Check sheet for the modelled part. Datum: model origin and axes. Units: mm. Face numbers are marked on the shaded views. Round coordinates to 2 decimals unless told otherwise and drop trailing zeros. Loops run counter-clockwise (first coordinate to the right, second up) from the corner with the lowest first, then second, coordinate; pieces in that order, holes last. Notation, with made-up numbers: (8.25, 65.25) - (64.25, 65.25) arc R33 ccw to (64.25, 96.25) - close; hole circle Ø9 at (44.5, -22.5). An arc over 180 degrees is marked (long way). Answer in a Markdown table with one row per item. Add a question column.
(1) Gauge pin test, flat ends, axial feed: pin 1 (3 mm diameter, centred on x = -10, y = 0, fed in from -Z); pin 2 (4.5 mm diameter, centred on x = 13, z = 21, fed in from +Y); pin 3 (10 mm diameter, centred on x = -2.5, z = 12.5, fed in from +Y). Record the tip position at first contact, or that the pin passes through.
(2) Cross-section at A-A on x = 13. Enter the section's corners in (y, z), then the cut area to 3 significant figures.
(3) Thickness scan on line 1 along Z through (x, y) = (-13, -4.05); line 2 along X through (y, z) = (-4.8, 9); line 3 along Z through (x, y) = (-13, -3.95). Record the ranges inside material, lowest first.
(4) Mould release check, pull along Y, two halves, no side actions. Record for the marked faces 1, 2, 3 and 4: +Y half, -Y half, draft (parallel to the pull), parting line (faces both ways), or undercut.
(5) Cross-section at C-C on z = 20.5. Enter the section's corners in (x, y).
(6) Cross-section at D-D on x = -2.5. Enter the section's corners in (y, z).
(7) Cross-section at B-B on y = 0. Enter the section's corners in (x, z), then the cut area to 3 significant figures.
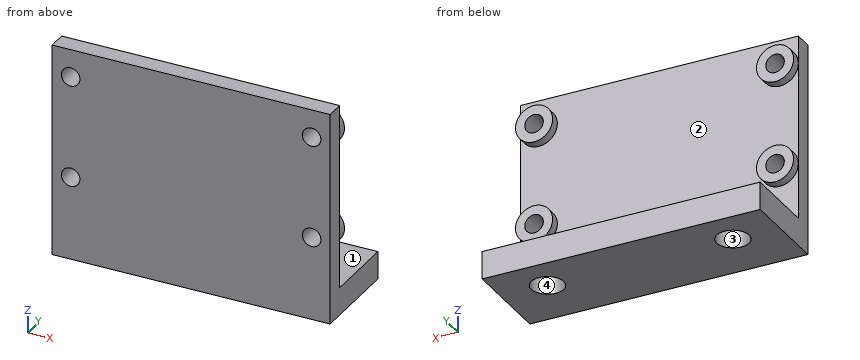
Autodesk Inventor part; units mm, degrees
ref_plane "YZ Plane" through (0, 0, 0) normal (1, 0, 0) x (0, 1, 0)
ref_plane "XZ Plane" through (0, 0, 0) normal (0, 1, 0) x (-1, 0, 0)
ref_plane "XY Plane" through (0, 0, 0) normal (0, 0, 1) x (1, 0, 0)
sketch "Sketch1" plane through (0, 0, 0) normal (0, 0, 1) x (1, 0, 0)
  circle A0 centre (-10, 0) radius 1.75
  circle A1 centre (10, 0) radius 1.75
  line L0 (-15, 4) -> (15, 4)
  line L1 (15, 4) -> (15, -6)
  line L2 (15, -6) -> (-15, -6)
  line L3 (-15, -6) -> (-15, 4)
  point P0 (0, 0)
  dimension "d0" = 10
  dimension "d1" = 10
  dimension "d2" = 3.5
  dimension "d3" = 5
  dimension "d4" = 5
  dimension "d5" = 4
  dimension "d6" = 10
extrude "Extrusion1" add sketch "Sketch1" along normal blind 3
sketch "Sketch2" plane through (0, 0, 3) normal (0, 0, 1) x (1, 0, 0)
  line L0 (-15, -6) -> (15, -6)
  line L1 (15, -6) -> (15, 4)
  line L2 (15, 4) -> (-15, 4)
  line L3 (-15, 4) -> (-15, -6)
  circle A0 centre (10, 0) radius 1.75
  circle A1 centre (-10, 0) radius 1.75
  line L4 (15, -6) -> (15, 4)
  line L5 (-15, -6) -> (15, -6)
  line L6 (15, -6) -> (15, -4)
  line L7 (15, -4) -> (-15, -4)
  line L8 (-15, -4) -> (-15, -6)
  point P0 (0, 0)
  dimension "d9" = 2
extrude "Extrusion2" add sketch "Sketch2" along normal blind 20 contours L3 L7 L1 L0
sketch "Sketch4" plane through (-15, -4, 3) normal (0, 1, 0) x (1, 0, 0)
  line L0 (0, 0) -> (30, 0)
  line L1 (0, 0) -> (0, -20)
  line L2 (30, -20) -> (0, -20)
  line L3 (30, 0) -> (30, -20)
  circle A0 centre (2, -6) radius 1
  circle A1 centre (28, -6) radius 1
  circle A2 centre (28, -17) radius 1
  circle A3 centre (2, -17) radius 1
  circle A4 centre (2, -6) radius 2
  line L4 (0, 3) -> (0, -20)
  circle A5 centre (2, -17) radius 2
  circle A6 centre (28, -17) radius 2
  line L5 (30, 3) -> (30, -20)
  circle A7 centre (28, -6) radius 2
  point P0 (15, 3)
  dimension "d12" = 2
  dimension "d13" = 26
  dimension "d14" = 11
  dimension "d15" = 2
  dimension "d16" = 6
extrude "Extrusion3" add sketch "Sketch4" along normal blind 1 contours A4 | A5 | A6 | A7
sketch "Sketch5" plane through (-13, -4, 9) normal (0, 1, 0) x (1, 0, 0)
  circle A0 centre (0, 0) radius 1
  circle A1 centre (26, 0) radius 1
  circle A2 centre (26, -11) radius 1
  circle A3 centre (0, -11) radius 1
  point P0 (13, 9)
extrude "Extrusion4" cut sketch "Sketch5" against normal through all
equation "\"d4\" = d3"
properties part number "Nozzlecam_PCB_Mount" material "ABS Plastic"
Answers:
| question | item | result |
|---|---|---|
| 1 | pin 1 | passes through |
| 1 | pin 2 | stops at y = -3 |
| 1 | pin 3 | stops at y = -4 |
| 2 | outline | (-6, 0) - (4, 0) - (4, 3) - (-4, 3) - (-4, 7) - (-3, 7) - (-3, 8) - (-6, 8) - close; (-6, 10) - (-3, 10) - (-3, 11) - (-4, 11) - (-4, 18) - (-3, 18) - (-3, 19) - (-6, 19) - close; (-6, 21) - (-3, 21) - (-3, 22) - (-4, 22) - (-4, 23) - (-6, 23) - close |
| 2 | area | 66.0 mm^2 |
| 3 | line 1 | z = 0 to 8, 10 to 19, 21 to 23 |
| 3 | line 2 | x = -15 to -14, -12 to 12, 14 to 15 |
| 3 | line 3 | z = 0 to 3, 7 to 8, 10 to 11, 18 to 19, 21 to 22 |
| 4 | face 1 | draft |
| 4 | face 2 | +Y half |
| 4 | face 3 | undercut |
| 4 | face 4 | undercut |
| 5 | outline | (-15, -6) - (-13.87, -6) - (-13.87, -3) - (-14.94, -3) - (-14.94, -4) - (-15, -4) - close; (-12.13, -6) - (12.13, -6) - (12.13, -3) - (11.06, -3) - (11.06, -4) - (-11.06, -4) - (-11.06, -3) - (-12.13, -3) - close; (13.87, -6) - (15, -6) - (15, -4) - (14.94, -4) - (14.94, -3) - (13.87, -3) - close |
| 6 | outline | (-6, 0) - (4, 0) - (4, 3) - (-4, 3) - (-4, 23) - (-6, 23) - close |
| 7 | outline | (-15, 0) - (-11.75, 0) - (-11.75, 3) - (-15, 3) - close; (-8.25, 0) - (8.25, 0) - (8.25, 3) - (-8.25, 3) - close; (11.75, 0) - (15, 0) - (15, 3) - (11.75, 3) - close |
| 7 | area | 69.0 mm^2 |
